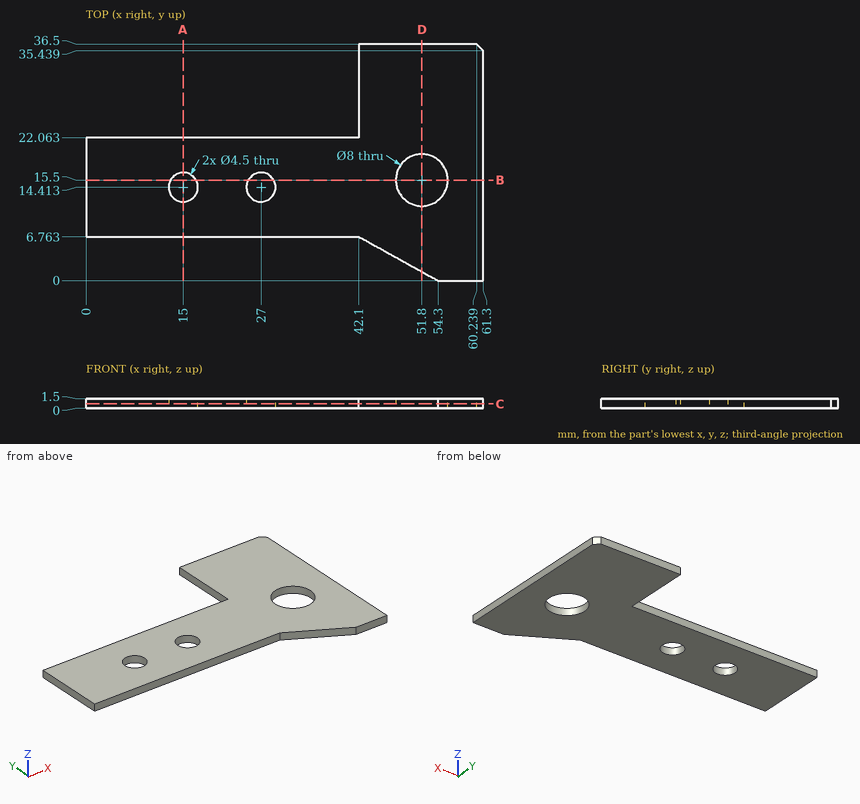
Could you check a few things on this drawing? It's one solid part, dimensions in mm from its lowest x, y, z. Coordinates: 2 decimals unless noted, no trailing zeros. Order: outer loops, then holes, each group sorted by start corner. A loop starts at its lowest first (then second) coordinate and runs counter-clockwise, first axis right, second up. Notation, with made-up numbers: (-3, 46.5) - (26, 46.5) arc R16 ccw to (26, 56.5) - close; hole circle Ø4 at (5.5, 2). An arc over 180 degrees is marked (long way). One line per question, with ' | ' between items.
(1) Will this pin go through, and if not, where does the flat tip stop? pin 1 (0.8 mm diameter, centred on y = 26.5, z = 0.5, fed in from -X).
Report:
pin 1: stops at x = 42.1
(2) Suppose I cut it at D-D on x = 51.8. List the corners of the cut face in (y, z) for me (1 decimal).
Report:
outline: (1.4, 0) - (11.5, 0) - (11.5, 1.5) - (1.4, 1.5) - close; (19.5, 0) - (36.5, 0) - (36.5, 1.5) - (19.5, 1.5) - close
(3) Suppose I cut it at C-C on z = 0.7. List the corners of the cut face in (x, y) for me.
Report:
outline: (0, 6.76) - (42.1, 6.76) - (54.3, 0) - (61.3, 0) - (61.3, 35.44) - (60.24, 36.5) - (42.1, 36.5) - (42.1, 22.06) - (0, 22.06) - close; hole circle Ø4.5 at (15, 14.41); hole circle Ø4.5 at (27, 14.41); hole circle Ø8 at (51.8, 15.5)
(4) Suppose I cut it at B-B on y = 15.5. List the corners of the cut face in (x, z) for me.
Report:
outline: (0, 0) - (13.03, 0) - (13.03, 1.5) - (0, 1.5) - close; (16.97, 0) - (25.03, 0) - (25.03, 1.5) - (16.97, 1.5) - close; (28.97, 0) - (47.8, 0) - (47.8, 1.5) - (28.97, 1.5) - close; (55.8, 0) - (61.3, 0) - (61.3, 1.5) - (55.8, 1.5) - close
(5) If I drill on L1, parallel to Y at x = 27, z = 0.6; L2, parallel to X at y = 16, z = 0.4 (1 decimal); L3, parallel to X at y = 28.5, z = 1.35, over which ranges is the centre line in solid material (lowest first)?
Report:
L1: y = 6.76 to 12.16, 16.66 to 22.06 | L2: x = 0 to 13.4, 16.6 to 25.4, 28.6 to 47.8, 55.8 to 61.3 | L3: x = 42.1 to 61.3
(6) Suppose I cut it at A-A on x = 15. List the corners of the cut face in (y, z) for me, and give its area (3 significant figures).
Report:
outline: (6.76, 0) - (12.16, 0) - (12.16, 1.5) - (6.76, 1.5) - close; (16.66, 0) - (22.06, 0) - (22.06, 1.5) - (16.66, 1.5) - close | area: 16.2 mm2
